Could you check a few things on this model? Use its own coordinates, in mm. Round coordinates to 2 decimals unless told otherwise and drop trailing zeros. Write each loop counter-clockwise with the first axis right and the second up, starting at its lowest first coordinate (ties: lowest second). Pieces come first, ordered by that corner, then holes. Notation, with made-up numbers: (53.5, -17) -> (89.5, -17) arc R13 cw to (89.5, -1) -> close; hole circle Ø10 at (68, -33). An arc over 180 degrees is marked (long way). Return JSON: item names as keys, results as strings.
Autodesk Fusion 360 part; units mm, degrees
sketch "3D-printed conduit top outline" plane through (0, 0, 0) normal (0, 1, 0) x (1, 0, 0)
  line L0 (0, 0) -> (16, 0)
  line L1 (16, 0) -> (16, -2)
  line L2 (16, -2) -> (0, -2)
  line L3 (0, -2) -> (0, 0)
  dimension "d7" = 16
  dimension "d8" = 2
extrude "Extrude1" add sketch "3D-printed conduit top outline" along normal blind 69.355
sketch "Magnet holes" plane through (0, 0, 2) normal (0, 0, 1) x (-1, 0, 0)
  line L0 (0, 0) -> (-16, 0)
  line L1 (-16, 0) -> (-16, -69.355)
  line L2 (-16, -69.355) -> (0, -69.355)
  line L3 (0, -69.355) -> (0, 0)
  circle A0 centre (-2.5, -2.5) radius 2.5
  circle A1 centre (-13.5, -2.5) radius 2.5
  circle A2 centre (-2.5, -2.5) radius 1.75
  circle A3 centre (-13.5, -2.5) radius 1.75
  circle A4 centre (-2.5, -66.855) radius 1.75
  circle A5 centre (-2.5, -66.855) radius 2.5
  circle A6 centre (-13.5, -50.855) radius 2.5
  circle A7 centre (-13.5, -50.855) radius 1.75
  dimension "d11" = 5
  dimension "d12" = 5
  dimension "d13" = 3.5
  dimension "d14" = 3.5
  dimension "d17" = 0
  dimension "d18" = -64.355
  dimension "d32" = 0
  dimension "d33" = -48.355
extrude "Extrude4" cut sketch "Magnet holes" against normal blind 1 contours A2 | A3 | A4 | A7
sketch "Support rib" plane through (0, 0, 2) normal (0, 0, 1) x (-1, 0, 0)
  circle A0 centre (-13.5, -2.5) radius 1.75
  circle A1 centre (-2.5, -66.855) radius 1.75
  circle A2 centre (-2.5, -2.5) radius 1.75
  circle A3 centre (-13.5, -50.855) radius 1.75
  line L0 (0, 0) -> (-16, 0)
  line L1 (-16, 0) -> (-16, -69.355)
  line L2 (-16, -69.355) -> (0, -69.355)
  line L3 (0, -69.355) -> (0, 0)
  line L4 (-5.5, 0) -> (-10.5, 0)
  line L5 (-10.5, 0) -> (-10.5, -65.355)
  line L6 (-10.5, -65.355) -> (-5.5, -65.355)
  line L7 (-5.5, -65.355) -> (-5.5, 0)
  dimension "d36" = 5
  dimension "d37" = 5.5
  dimension "d38" = 5.5
  dimension "d39" = 4
extrude "Extrude3" add sketch "Support rib" along normal blind 3 contours L0 L4 L5 L6 L7
chamfer "Chamfer2" distance 0.5 angle 45 2 edges at (10.5, 32.6775, 5) (5.5, 32.6775, 5)
equation "conduit_length = 69.355 mm"
equation "conduit_width = 16 mm"
equation "conduit_wall_thickness = 2 mm"
equation "magnet_diameter = 3 mm"
equation "magnet_height = 1 mm"
equation "d7 = conduit_width"
equation "d8 = conduit_wall_thickness"
equation "d9 = conduit_length"
equation "d11 = magnet_diameter + 2 mm"
equation "d12 = magnet_diameter + 2 mm"
equation "d13 = magnet_diameter + 0.5 mm"
equation "d14 = magnet_diameter + 0.5 mm"
equation "d18 = -conduit_length + ( magnet_diameter + 2 mm )"
equation "rib_width = 5 mm"
equation "rib_height = 3 mm"
equation "d26 = rib_height"
equation "rib_chamfer = 0.5 mm"
equation "d33 = -conduit_length + ( magnet_diameter + 2 mm ) + ( conduit_width )"
equation "d36 = rib_width"
equation "d37 = ( conduit_width - rib_width ) / 2"
equation "d39 = 2 * conduit_wall_thickness"
equation "d40 = rib_chamfer"
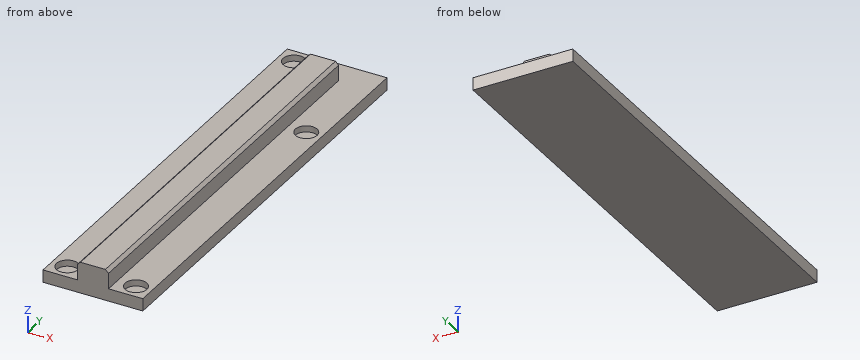
1) Will these pins go through, and if not, where does the flat tip stop? pin 1 Ø4.5 at (x, y) = (13.5, 2.5) entering from +Z; pin 2 Ø2 at (y, z) = (41.5, 3.5) entering from -X; pin 3 Ø2 at (x, z) = (8, 3.5) entering from +Y (3 decimals).
Return value:
{"pin 1": "z = 2", "pin 2": "x = 5.5", "pin 3": "y = 65.355"}
2) I want a section at C-C, the plane z = 2.75. Please give me the cut outline in (x, y) (3 decimals).
Return value:
{"outline": "(5.5, 0) -> (10.5, 0) -> (10.5, 65.355) -> (5.5, 65.355) -> close"}
3) If I drill on probe 1 along Y at (x, z) = (2.5, 1.65) (3 decimals); probe 2 along Y at (x, z) = (13.5, 1.35) (3 decimals); probe 3 along Z at (x, y) = (11, 17.5), over which ranges is the centre line in solid material (lowest first)? Write a range as [from, to].
Return value:
{"probe 1": "[0, 0.75], [4.25, 65.105], [68.605, 69.355]", "probe 2": "[0, 0.75], [4.25, 49.105], [52.605, 69.355]", "probe 3": "[0, 2]"}
4) I want a section at A-A, the plane x = 13.5. Please give me the cut outline in (y, z) (3 decimals), and give its area (3 significant figures).
Return value:
{"outline": "(0, 0) -> (69.355, 0) -> (69.355, 2) -> (52.605, 2) -> (52.605, 1) -> (49.105, 1) -> (49.105, 2) -> (4.25, 2) -> (4.25, 1) -> (0.75, 1) -> (0.75, 2) -> (0, 2) -> close", "area": "132 mm²"}
5) I want a section at B-B, the plane y = 38.5. Please give me the cut outline in (x, z), and give its area (4 significant figures).
Return value:
{"outline": "(0, 0) -> (16, 0) -> (16, 2) -> (10.5, 2) -> (10.5, 4.5) -> (10, 5) -> (6, 5) -> (5.5, 4.5) -> (5.5, 2) -> (0, 2) -> close", "area": "46.75 mm²"}
6) I want a section at D-D, the plane x = 7.25. Please give me the cut outline in (y, z) (3 decimals), and give its area (3 significant figures).
Return value:
{"outline": "(0, 0) -> (69.355, 0) -> (69.355, 2) -> (65.355, 2) -> (65.355, 5) -> (0, 5) -> close", "area": "335 mm²"}
